Check sheet for the modelled part. Datum: model origin and axes. Units: mm. A direction names the side the tool comes from. Coordinates: 2 decimals unless noted, no trailing zeros. Loops run counter-clockwise (first coordinate to the right, second up) from the corner with the lowest first, then second, coordinate; pieces in that order, holes last.
from build123d import *

# Parameters (mm, degrees)
SKETCH1_W                     = 50
SKETCH1_H                     = 7
REVOLVE5_ANGLE                = 167.5
SHELL2_T                      = 3
CUT_EXTRUDE3_DEPTH            = 77.072333999
CUT_EXTRUDE3_DEPTH_BACK       = 10
CUT_EXTRUDE4_DEPTH            = 77.072333999
CUT_EXTRUDE4_DEPTH_BACK       = 10
CUT_EXTRUDE_THIN1_DEPTH       = 77.072333999
CUT_EXTRUDE_THIN1_DEPTH_BACK  = 20
CUT_EXTRUDE_THIN2_DEPTH       = 77.072333999
CUT_EXTRUDE_THIN2_DEPTH_BACK  = 20
CUT_EXTRUDE_THIN3_DEPTH       = 76.000787866
CUT_EXTRUDE_THIN3_DEPTH_BACK  = 20
SKETCH18_R                    = 8
BOSS_EXTRUDE3_DEPTH           = 3
CUT_EXTRUDE_THIN11_DEPTH      = 76.000787866
CUT_EXTRUDE_THIN11_DEPTH_BACK = 20
CUT_EXTRUDE_THIN12_DEPTH      = 76.000787866
CUT_EXTRUDE_THIN12_DEPTH_BACK = 20
FILLET2_R                     = 40


with BuildPart() as part:
    # Sketch1 → Revolve5 (revolve)
    with BuildSketch(Plane(origin=(0, 0, 0), x_dir=(1, 0, 0), z_dir=(0, 1, 0))):
        with Locations((25, 3.5)):
            Rectangle(SKETCH1_W, SKETCH1_H)
    revolve(axis=Axis((0, 0, 0), (0, 0, 1)), revolution_arc=REVOLVE5_ANGLE)

    # Shell2
    shell2_openings = [part.faces().sort_by_distance(p)[0] for p in [
        (25, 0, -3.5),
        (-24.407400178, 5.410990348, -3.5),
    ]]
    offset(amount=SHELL2_T, openings=shell2_openings, kind=Kind.INTERSECTION)

    # Sketch11 → Cut-Extrude3 (cut, two sides: drawn at the far end of the back side and taken through both)
    with BuildSketch(Plane.XY.offset(3).offset(-CUT_EXTRUDE3_DEPTH_BACK)):
        Polygon((-295.067343662, 38.119573796), (-51.743688377, 11.471299539), (53, 0), (296.323655284, -26.648274258), (243.027106769, -513.295584826), (-348.363892177, -448.527736772), align=None)
    extrude(amount=CUT_EXTRUDE3_DEPTH + CUT_EXTRUDE3_DEPTH_BACK, mode=Mode.SUBTRACT)

    # Sketch12 → Cut-Extrude4 (cut, two sides: drawn at the far end of the back side and taken through both)
    with BuildSketch(Plane(origin=(0, 0, -10), x_dir=(-1, 0, 0), z_dir=(0, 0, -1)).offset(-CUT_EXTRUDE4_DEPTH_BACK)):
        Polygon((-296.323655284, -26.648274258), (-53, 0), (51.743688377, 11.471299539), (295.067343662, 38.119573796), (348.363892177, -448.527736772), (-243.027106769, -513.295584826), align=None)
    extrude(amount=CUT_EXTRUDE4_DEPTH + CUT_EXTRUDE4_DEPTH_BACK, mode=Mode.SUBTRACT)

    # Sketch13 → Cut-Extrude-Thin1 (cut, two sides: drawn at the far end of the back side and taken through both)
    with BuildSketch(Plane(origin=(0, 0, -10), x_dir=(-1, 0, 0), z_dir=(0, 0, -1)).offset(-CUT_EXTRUDE_THIN1_DEPTH_BACK)):
        Polygon((48.779244367, 11.146640118), (47.419699991, 23.560551191), (57.360263374, 24.64921994), (58.719807749, 12.235308866), align=None)
    extrude(amount=CUT_EXTRUDE_THIN1_DEPTH + CUT_EXTRUDE_THIN1_DEPTH_BACK, mode=Mode.SUBTRACT)

    # Sketch14 → Cut-Extrude-Thin2 (cut, two sides: drawn at the far end of the back side and taken through both)
    with BuildSketch(Plane(origin=(0, 0, -10), x_dir=(-1, 0, 0), z_dir=(0, 0, -1)).offset(-CUT_EXTRUDE_THIN2_DEPTH_BACK)):
        Polygon((-50.035555989, 0.324659421), (-51.39409796, 12.729417605), (-81.215788107, 9.46341136), (-79.857246136, -2.941346825), align=None)
    extrude(amount=CUT_EXTRUDE_THIN2_DEPTH + CUT_EXTRUDE_THIN2_DEPTH_BACK, mode=Mode.SUBTRACT)

    # Sketch15 → Cut-Extrude-Thin3 (cut, two sides: drawn at the far end of the back side and taken through both)
    with BuildSketch(Plane(origin=(0, 0, -10), x_dir=(-1, 0, 0), z_dir=(0, 0, -1)).offset(-CUT_EXTRUDE_THIN3_DEPTH_BACK)):
        with BuildLine():
            ThreePointArc((-41.982664634, 1.20659446), (-4.572408744, 41.750366205), (40.726353012, 10.264705079))
            Line((40.726353012, 10.264705079), (11.636100861, 2.93277288))
            ThreePointArc((11.636100861, 2.93277288), (-1.306402498, 11.928676059), (-11.995047038, 0.344741274))
            Line((-11.995047038, 0.344741274), (-41.982664634, 1.20659446))
        make_face()
    extrude(amount=CUT_EXTRUDE_THIN3_DEPTH + CUT_EXTRUDE_THIN3_DEPTH_BACK, mode=Mode.SUBTRACT)


with BuildPart() as body_2:
    # of the pieces the cut leaves, the one that is kept (cut_extrude_thin3_keep)
    add(part.part.solids().sort_by_distance((49.998919737, 0.328671743, 0))[0])

    # Sketch18 → Boss-Extrude3 (add)
    with BuildSketch(Plane.XY.offset(3)):
        with Locations((-39.855418013, 18.217155785)):
            Circle(SKETCH18_R)
        with Locations((42.853599633, 9.159045166)):
            Circle(SKETCH18_R)
    extrude(amount=-BOSS_EXTRUDE3_DEPTH)

    # Sketch26 → Cut-Extrude-Thin11 (cut, two sides: drawn at the far end of the back side and taken through both)
    with BuildSketch(Plane.XY.offset(3).offset(-CUT_EXTRUDE_THIN11_DEPTH_BACK)):
        with BuildLine():
            ThreePointArc((-48.779244367, 11.146640118), (-44.869380897, 25.502903795), (-36.885486711, 38.058650397))
            Line((-36.885486711, 38.058650397), (-51.966031339, 51.195513559))
            ThreePointArc((-51.966031339, 51.195513559), (-63.162508763, 33.587548061), (-68.645634797, 13.454568038))
            Line((-68.645634797, 13.454568038), (-48.779244367, 11.146640118))
        make_face()
    extrude(amount=CUT_EXTRUDE_THIN11_DEPTH + CUT_EXTRUDE_THIN11_DEPTH_BACK, mode=Mode.SUBTRACT)

    # Sketch27 → Cut-Extrude-Thin12 (cut, two sides: drawn at the far end of the back side and taken through both)
    with BuildSketch(Plane.XY.offset(3).offset(-CUT_EXTRUDE_THIN12_DEPTH_BACK)):
        with BuildLine():
            ThreePointArc((50.035555989, 0.324659421), (49.325636064, 15.186871666), (44.248552996, 29.173027916))
            Line((44.248552996, 29.173027916), (61.814966092, 38.73446771))
            ThreePointArc((61.814966092, 38.73446771), (68.93498104, 19.120520049), (69.93056067, -1.721993641))
            Line((69.93056067, -1.721993641), (50.035555989, 0.324659421))
        make_face()
    extrude(amount=CUT_EXTRUDE_THIN12_DEPTH + CUT_EXTRUDE_THIN12_DEPTH_BACK, mode=Mode.SUBTRACT)

    # Fillet2
    # the kernel refuses this fillet: 40 mm, written as the material it takes off along each edge
    with BuildSketch(Plane(origin=(-36.885486711, 38.058650397, -30.526100609), x_dir=(-0.5923211564074143, -0.8057019595807023, 0), z_dir=(0, 0, 1)), Plane(origin=(44.248552996, 29.173027916, 23.526100609), x_dir=(0.4038949588524026, -0.9148053684875357, 0), z_dir=(0, 0, -1))) as fillet2_piece_1:
        with BuildLine():
            CenterArc((4.906698725, 39.863332675), FILLET2_R, 252.499995648, 22.237662415)
            ThreePointArc((-7.121536153, 1.714655559), (-3.59042601, 0.734148493), (0, 0))
            ThreePointArc((0, 0), (4.105220122, -0.169822442), (8.210440244, 0))
        make_face()
    extrude(amount=54.052201219, mode=Mode.SUBTRACT)


solid = body_2.part
(1) Gauge pin test, flat ends, axial feed: P1, Ø3, axis at x = 11.5, z = 0.5, coming from the -Y side; P2, Ø5, axis at x = 24.5, z = -7.5, coming from the +Y side; P3, Ø5, axis at y = 25.5, z = -6.5, coming from the -X side. Record the tip position at first contact, or that the pin passes through.
(2) Draft check along Y on faces 1 (the face through (35.002, 7.624, 1.521)), 2 (the face through (49.984, 10.978, -3.591)), 3 (the face through (46.07, 0.76, -7.92)). Enter one of: pulls with the +Y half, pulls with the -Y half, needs draft (parallel to the pull), parting line crosses it, or undercut.
(3) Section check A-A, the plane y = 26. Enter the section's corners in (x, z).
(4) Scan lines: line 1 along Z through (x, y) = (-28.5, 32); line 2 along Z through (x, y) = (-38.5, 12.5); line 3 along X through (y, z) = (25, -6.25). Record each from-to range of solid material in increasing order.
(5) Section check D-D, the plane y = 48.5. Enter the section's corners in (x, z).
(6) Set-up check for faces 4 (the face through (4, 42, 0)), 5 (the face through (-46.42, 21.54, -3.59)), 6 (the face through (5.41, 41.65, -8.48)): record each of +Z, -Z, +X, -X, +Y, -Y from which the full face is reachable in a straight line by a thin tool's end or side.
(7) Section check B-B, the plane x = 0. Enter the section's corners in (y, z), plus the area to 3 significant figures.
(8) Section check C-C, the plane z = -8.5. Enter the section's corners in (x, y), plus the area to 3 significant figures.
Determined:
1. P1: stops at y = 39.94
1. P2: stops at y = 48.22
1. P3: stops at x = -45.9
2. face 1: undercut
2. face 2: parting line crosses it
2. face 3: pulls with the -Y half
3. outline: (-44.65, -10) - (-32.98, -10) - (-32.98, -7) - (-42.71, -7) - (-42.71, 0) - (-32.98, 0) - (-32.98, 3) - (-44.65, 3) - close; (32.98, -10) - (45.77, -10) - (45.77, 3) - (32.98, 3) - (32.98, 0) - (42.71, 0) - (42.71, -7) - (32.98, -7) - close
4. line 1: z = -10 to -7, 0 to 3
4. line 2: z = 0 to 3
4. line 3: x = -45.09 to -43.3, 43.3 to 46.24
5. outline: (-21.37, -10) - (21.37, -10) - (21.37, 3) - (-21.37, 3) - close; hole (-12.16, -7) - (12.16, -7) - (12.16, 0) - (-12.16, 0) - close
6. face 4: -Y
6. face 5: +Z, -Z, -X, +Y
6. face 6: -Z, -Y
7. outline: (42, -10) - (53, -10) - (53, 3) - (42, 3) - (42, 0) - (50, 0) - (50, -7) - (42, -7) - close
7. area: 87.0 mm2
8. outline: (-48.78, 11.15) - (-40.73, 10.26) arc R42 cw to (41.98, 1.21) - (50.04, 0.32) arc R49.7 ccw to (47.56, 21.66) arc R40 ccw to (39.8, 35) arc R53 ccw to (-31.29, 42.78) arc R40 ccw to (-41.75, 31.44) arc R49.7 ccw to start
8. area: 1,430 mm2
